```python
from build123d import *

# Parameters (mm, degrees)
SKETCH1_W           = 25
SKETCH1_H           = 30
BOSS_EXTRUDE1_DEPTH = 5
CUT_EXTRUDE1_DEPTH  = 0.3
SKETCH3_R           = 1.85
BOSS_EXTRUDE2_DEPTH = 2.5
FILLET3_R           = 2.5
SKETCH2_3_R         = 2.6
CUT_EXTRUDE7_DEPTH  = 10
SKETCH2_4_R         = 4.6
CUT_EXTRUDE8_DEPTH  = 1.5
FILLET4_R           = 0.5


with BuildPart() as part:
    # Sketch1 → Boss-Extrude1 (new body)
    with BuildSketch(Plane(origin=(0, 0, 0), x_dir=(1, 0, 0), z_dir=(0, 1, 0))):
        with Locations((12.5, 15)):
            Rectangle(SKETCH1_W, SKETCH1_H)
    extrude(amount=BOSS_EXTRUDE1_DEPTH)

    # Sketch2 → Cut-Extrude1 (cut)
    with BuildSketch(Plane(origin=(0, 5, 0), x_dir=(1, 0, 0), z_dir=(0, 1, 0))):
        with BuildLine():
            Line((8, 25), (17, 25))
            ThreePointArc((17, 25), (19.121320344, 24.121320344), (20, 22))
            Line((20, 22), (20, 12))
            ThreePointArc((20, 12), (19.805806757, 10.038838649), (19.230769231, 8.153846154))
            Line((19.230769231, 8.153846154), (19.519230769, 8.846153846))
            ThreePointArc((19.519230769, 8.846153846), (18.944193243, 6.961161351), (18.75, 5))
            Line((18.75, 5), (18.75, 0))
            Line((18.75, 0), (6.25, 0))
            Line((6.25, 0), (6.25, 5))
            ThreePointArc((6.25, 5), (6.055806757, 6.961161351), (5.480769231, 8.846153846))
            Line((5.480769231, 8.846153846), (5.769230769, 8.153846154))
            ThreePointArc((5.769230769, 8.153846154), (5.194193243, 10.038838649), (5, 12))
            Line((5, 12), (5, 22))
            ThreePointArc((5, 22), (5.878679656, 24.121320344), (8, 25))
        make_face()
    extrude(amount=-CUT_EXTRUDE1_DEPTH, mode=Mode.SUBTRACT)

    # Sketch3 → Boss-Extrude2 (add)
    with BuildSketch(Plane(origin=(0, 5, 0), x_dir=(1, 0, 0), z_dir=(0, 1, 0))):
        with Locations((21, 27)):
            Circle(SKETCH3_R)
        with Locations((4, 27)):
            Circle(SKETCH3_R)
        with Locations((3, 4)):
            Circle(SKETCH3_R)
        with Locations((22, 4)):
            Circle(SKETCH3_R)
    extrude(amount=BOSS_EXTRUDE2_DEPTH)

    # Fillet3
    fillet3_edges = [part.edges().sort_by_distance(p)[0] for p in [
        (25, 0, -15),
        (0, 0, -15),
    ]]
    fillet(fillet3_edges, radius=FILLET3_R)

    # Sketch2_3 → Cut-Extrude7 (cut)
    with BuildSketch(Plane(origin=(0, 5, 0), x_dir=(1, 0, 0), z_dir=(0, 1, 0))):
        with Locations((12.5, 16)):
            Circle(SKETCH2_3_R)
    extrude(amount=-CUT_EXTRUDE7_DEPTH, mode=Mode.SUBTRACT)

    # Sketch2_4 → Cut-Extrude8 (cut)
    with BuildSketch(Plane(origin=(0, 5, 0), x_dir=(1, 0, 0), z_dir=(0, 1, 0))):
        with Locations((12.5, 16)):
            Circle(SKETCH2_4_R)
    extrude(amount=-CUT_EXTRUDE8_DEPTH, mode=Mode.SUBTRACT)

    # Fillet4
    fillet4_edges = [part.edges().sort_by_distance(p)[0] for p in [
        (2.15, 7.5, -27),
        (19.15, 7.5, -27),
        (20.15, 7.5, -4),
        (1.15, 7.5, -4),
    ]]
    fillet(fillet4_edges, radius=FILLET4_R)


solid = part.part
```
Geometry check sheet. Reference: the model listing, model coordinates, mm. A direction names the side the tool comes from. Coordinates: 2 decimals unless noted, no trailing zeros. Loops run counter-clockwise (first coordinate to the right, second up) from the corner with the lowest first, then second, coordinate; pieces in that order, holes last.
Item 1: Release check for a two-part mould opening along X. For faces 3 (the face through (12, 2, -30)), 4 (the face through (24.248, 0.713, -15.21)), 5 (the face through (19.636, 5.986, -28.25)), 6 (the face through (3.759, 5.986, -28.834)) record: released by +X, released by -X, zero draft, split by the parting line, or undercut.
Item 2: Sectioned sample at C-C, the plane y = 3. Record the boundary of the cut face in (x, z).
Item 3: Sectioned sample at A-A, the plane x = 12.5. Record the boundary of the cut face in (y, z).
Item 4: Sectioned sample at B-B, the plane z = -16. Record the boundary of the cut face in (x, y), then the cut area to 3 significant figures.
Item 5: Go/stop test with flat-tipped pins: pin 1 Ø7.5 at (x, z) = (9, -9.5) entering from +Y; pin 2 Ø6 at (x, z) = (12.5, -16) entering from +Y; pin 3 Ø4 at (x, z) = (8, -11.5) entering from +Y. Record where each tip stops, or that it passes through.
Item 6: Thickness scan on line 1 (X direction, y = 4.75, z = -1.5); line 2 (X direction, y = 4.15, z = -16); line 3 (Z direction, x = 12.5, y = 1.05). Record the ranges inside material, lowest first.
Item 7: Sectioned sample at D-D, the plane z = -27. Record the boundary of the cut face in (x, y).
Item 8: Access from +Z, -Z, +X, -X, +Y, -Y to the whole of each face (thin tool, end or side, straight path). Record for faces 1 (the face through (14.9, 1.8, -15)), 2 (the face through (12.3, 5, -25.2)).
Check result:
1. face 3: zero draft
1. face 4: released by +X
1. face 5: undercut
1. face 6: undercut
2. outline: (0, -30) - (25, -30) - (25, 0) - (0, 0) - close; hole circle Ø5.2 at (12.5, -16)
3. outline: (0, -30) - (5, -30) - (5, -25) - (4.7, -25) - (4.7, -20.6) - (3.5, -20.6) - (3.5, -18.6) - (0, -18.6) - close; (0, -13.4) - (3.5, -13.4) - (3.5, -11.4) - (4.7, -11.4) - (4.7, 0) - (0, 0) - close
4. outline: (0, 2.5) arc R2.5 ccw to (2.5, 0) - (9.9, 0) - (9.9, 3.5) - (7.9, 3.5) - (7.9, 4.7) - (5, 4.7) - (5, 5) - (0, 5) - close; (15.1, 0) - (22.5, 0) arc R2.5 ccw to (25, 2.5) - (25, 5) - (20, 5) - (20, 4.7) - (17.1, 4.7) - (17.1, 3.5) - (15.1, 3.5) - close
4. area: 88.6 mm2
5. pin 1: stops at y = 5
5. pin 2: stops at y = 3.5
5. pin 3: stops at y = 4.7
6. line 1: x = 0 to 6.25, 18.75 to 25
6. line 2: x = 0 to 7.9, 17.1 to 25
6. line 3: z = -30 to -18.6, -13.4 to 0
7. outline: (0, 2.5) arc R2.5 ccw to (2.5, 0) - (22.5, 0) arc R2.5 ccw to (25, 2.5) - (25, 5) - (22.85, 5) - (22.85, 7) arc R0.5 ccw to (22.35, 7.5) - (19.65, 7.5) arc R0.5 ccw to (19.15, 7) - (19.15, 5) - (5.85, 5) - (5.85, 7) arc R0.5 ccw to (5.35, 7.5) - (2.65, 7.5) arc R0.5 ccw to (2.15, 7) - (2.15, 5) - (0, 5) - close
8. face 1: +Y, -Y
8. face 2: +Y
